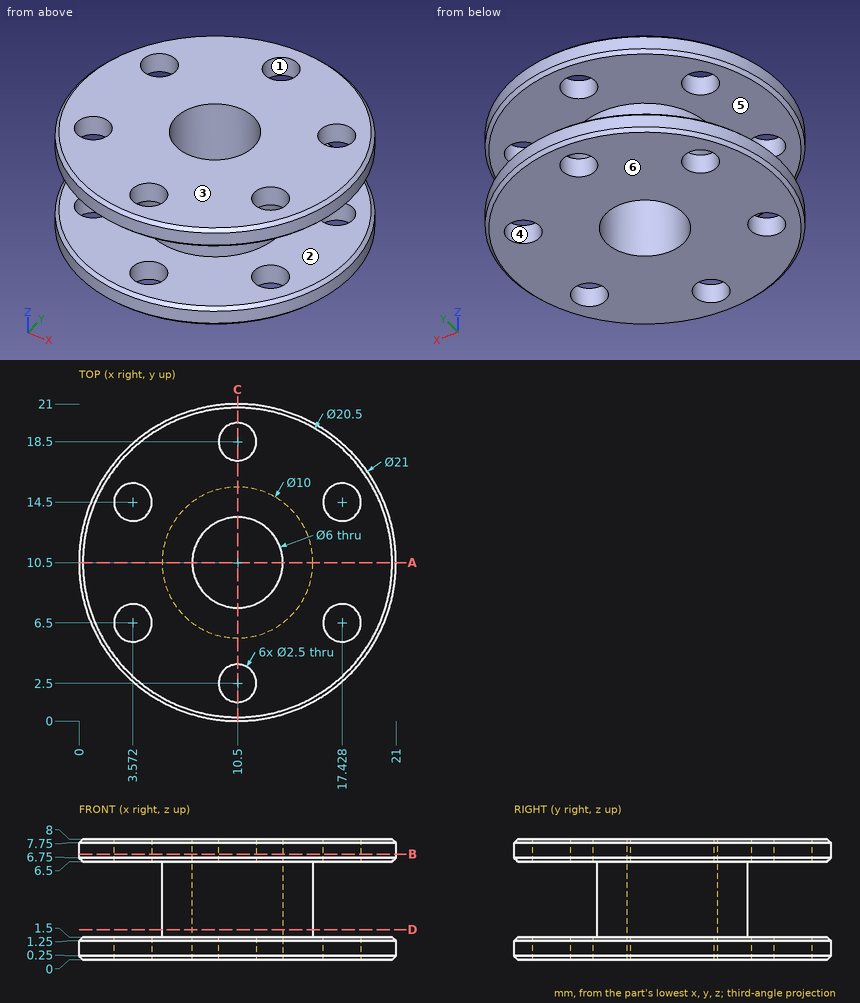
Design review of the part shown in the three views and the two pictorial views. Dimensions are in mm from the part's minimum x, y and z. A direction names the side the tool comes from. Round coordinates to 2 decimals unless told otherwise and drop trailing zeros. Loops run counter-clockwise (first coordinate to the right, second up) from the corner with the lowest first, then second, coordinate; pieces in that order, holes last. Notation, with made-up numbers: (-35, 31) - (-21, 31) arc R32 ccw to (-21, 59) - close; hole circle Ø3 at (-6.75, 12). An arc over 180 degrees is marked (long way). Answer as CSV lines item,"result".
(1) Consider section A-A on y = 10.5. Give the boundary of the cut face in (x, z).
Checked values:
outline,"(0, 0.25) - (0.25, 0) - (7.5, 0) - (7.5, 8) - (0.25, 8) - (0, 7.75) - (0, 6.75) - (0.25, 6.5) - (5.5, 6.5) - (5.5, 1.5) - (0.25, 1.5) - (0, 1.25) - close; (13.5, 0) - (20.75, 0) - (21, 0.25) - (21, 1.25) - (20.75, 1.5) - (15.5, 1.5) - (15.5, 6.5) - (20.75, 6.5) - (21, 6.75) - (21, 7.75) - (20.75, 8) - (13.5, 8) - close"
(2) Consider section B-B on z = 7. Give the boundary of the cut face in (x, y).
Checked values:
outline,"circle Ø21 at (10.5, 10.5); hole circle Ø2.5 at (3.57, 6.5); hole circle Ø2.5 at (3.57, 14.5); hole circle Ø6 at (10.5, 10.5); hole circle Ø2.5 at (10.5, 2.5); hole circle Ø2.5 at (10.5, 18.5); hole circle Ø2.5 at (17.43, 6.5); hole circle Ø2.5 at (17.43, 14.5)"
(3) Insertion check: P1, Ø3, axis at x = 3.57, y = 6.5, coming from the -Z side; P2, Ø1, axis at x = 15.5, z = 1, coming from the +Y side. Each pin has a flat end and moves straight along its axis. Give the tip position at first contact, or say it passes through.
Checked values:
P1,"stops at z = 0"
P2,"stops at y = 19.99"
(4) Mouldability with a two-part tool opening along Z and no side actions: class the marked faces 3, 4, 5 and 6 as +Z half, -Z half, draft (parallel to the pull), parting line (faces both ways), or undercut.
Checked values:
face 3,"+Z half"
face 4,"draft"
face 5,"undercut"
face 6,"-Z half"
(5) Wall thickness on line 1 (Y direction, x = 10.5, z = 7.6); line 2 (Z direction, x = 4.75, y = 2.5); line 3 (Y direction, x = 10.5, z = 5.5): over which ranges is each line inside the solid? List them lowest first.
Checked values:
line 1,"y = 0 to 1.25, 3.75 to 7.5, 13.5 to 17.25, 19.75 to 21"
line 2,"z = 0 to 1.5, 6.5 to 8"
line 3,"y = 5.5 to 7.5, 13.5 to 15.5"
(6) Consider section D-D on z = 2. Give the boundary of the cut face in (x, y).
Checked values:
outline,"circle Ø10 at (10.5, 10.5); hole circle Ø6 at (10.5, 10.5)"
(7) Consider section C-C on x = 10.5. Give the number of separate pieces and of enclosed holes in the cut face.
Checked values:
separate pieces,"6"
enclosed holes,"0"
(8) Tool access review of the marked faces 1 and 2: name each direction out of +Z, -Z, +X, -X, +Y, -Y from which nothing blocks a thin tool from reaching the whole face with its end or side.
Checked values:
face 1,"+Z, -Z"
face 2,"none"
